Here's how the part is built. I have some questions about the finished solid (model axes, mm). A direction names the side the tool comes from. Coordinates: 2 decimals unless noted, no trailing zeros. Write each loop counter-clockwise with the first axis right and the second up, starting at its lowest first coordinate (ties: lowest second). Pieces come first, ordered by that corner, then holes. Notation, with made-up numbers: (39, 26) -> (46, 26) arc R27 ccw to (46, 65) -> close; hole circle Ø7 at (35, 74). An arc over 180 degrees is marked (long way). Use a Markdown table: item, result. Add a question column.
```python
from build123d import *

# Parameters (mm, degrees)
BODY_DEPTH             = 10
SKETCH14_R             = 7.5
BEARING_SUPPORT_DEPTH  = 15
SKETCH15_R             = 7.5
SKETCH15_R_2           = 4.7
BEARING_PLACE_DEPTH    = 4
SKETCH16_R             = 2
MOTOR_SHAFT_HOLE_DEPTH = 3
FILLET1_R              = 6
SKETCH17_R             = 7.25
SPRING_HOLE_DEPTH      = 10
SKETCH18_W             = 11
SKETCH18_H             = 6
NUT_HOLE_DEPTH         = 20
SKETCH19_R             = 3.25
SHAFT_HOLE_DEPTH       = 13
SKETCH20_R             = 3.25
BRAKE_DISK_HOLES_DEPTH = 67.708320321


with BuildPart() as part:
    # Sketch1 → Body (new, symmetric)
    with BuildSketch(Plane.XY):
        Polygon((-25, 25), (-15, 45), (15, 45), (25, 25), (25, 5), (45, 5), (45, -25), (25, -25), (-25, -25), (-45, -25), (-45, 5), (-25, 5), align=None)
    extrude(amount=BODY_DEPTH, both=True)

    # Sketch14 → Bearing_Support (add)
    with BuildSketch(Plane(origin=(0, 0, -10), x_dir=(-1, 0, 0), z_dir=(0, 0, -1))):
        Circle(SKETCH14_R)
    extrude(amount=BEARING_SUPPORT_DEPTH)

    # Sketch15 → Bearing_Place (add)
    with BuildSketch(Plane(origin=(0, 0, -25), x_dir=(-1, 0, 0), z_dir=(0, 0, -1))):
        Circle(SKETCH15_R)
        Circle(SKETCH15_R_2, mode=Mode.SUBTRACT)
    extrude(amount=BEARING_PLACE_DEPTH)

    # Sketch16 → Motor_Shaft_Hole (cut)
    with BuildSketch(Plane(origin=(0, 0, -25), x_dir=(-1, 0, 0), z_dir=(0, 0, -1))):
        Circle(SKETCH16_R)
    extrude(amount=-MOTOR_SHAFT_HOLE_DEPTH, mode=Mode.SUBTRACT)

    # Fillet1
    fillet1_edges = [part.edges().sort_by_distance(p)[0] for p in [
        (7.5, 0, -10),
    ]]
    fillet(fillet1_edges, radius=FILLET1_R)

    # Sketch17 → Spring_Hole (cut)
    with BuildSketch(Plane(origin=(0, 5, 0), x_dir=(1, 0, 0), z_dir=(0, 1, 0))):
        with Locations(Location((-35, 0, 0), (0, 0, 180))):
            Circle(SKETCH17_R)
    spring_hole = extrude(amount=-SPRING_HOLE_DEPTH, mode=Mode.SUBTRACT)

    # Sketch18 → Nut_Hole (cut)
    with BuildSketch(Plane.ZY.offset(45)):
        with Locations((0, -15)):
            Rectangle(SKETCH18_W, SKETCH18_H)
    nut_hole = extrude(amount=-NUT_HOLE_DEPTH, mode=Mode.SUBTRACT)

    # Sketch19 → Shaft_Hole (cut)
    with BuildSketch(Plane(origin=(0, -5, 0), x_dir=(1, 0, 0), z_dir=(0, 1, 0))):
        with Locations(Location((-35, 0, 0), (0, 0, 180))):
            Circle(SKETCH19_R)
    shaft_hole = extrude(amount=-SHAFT_HOLE_DEPTH, mode=Mode.SUBTRACT)

    # Mirror1: Spring_Hole, Nut_Hole, Shaft_Hole across plane
    add(spring_hole.mirror(Plane(origin=(0, 0, 0), x_dir=(0, 0, 1), z_dir=(1, 0, 0))), mode=Mode.SUBTRACT)
    add(nut_hole.mirror(Plane(origin=(0, 0, 0), x_dir=(0, 0, 1), z_dir=(1, 0, 0))), mode=Mode.SUBTRACT)
    add(shaft_hole.mirror(Plane(origin=(0, 0, 0), x_dir=(0, 0, 1), z_dir=(1, 0, 0))), mode=Mode.SUBTRACT)

    # Sketch20 → Brake_Disk_Holes (cut, through all)
    with BuildSketch(Plane(origin=(0, 0, -10), x_dir=(-1, 0, 0), z_dir=(0, 0, -1))):
        with Locations((-5.98239088, 24.273668848)):
            Circle(SKETCH20_R)
        with Locations((24.012809306, -6.955931947)):
            Circle(SKETCH20_R)
        with Locations((-18.030418426, -17.317736902)):
            Circle(SKETCH20_R)
    extrude(amount=-BRAKE_DISK_HOLES_DEPTH, mode=Mode.SUBTRACT)


solid = part.part
```
Q1. Which directions (+Z, -Z, +X, -X, +Y, -Y) give clear straight access to the entire face, cutting with the end or side of a thin tool? Please do faces 3 (the cylindrical face through (38.002, -8.451, -1.245)), 4 (the cylindrical face through (7.493, 0.33, -22.409)), 5 (the flat face through (35, -15, -5.5)), 6 (the flat face through (28, 5, 5)), 7 (the flat face through (-37, -12, -3)).
Q2. Please list where these lines run through material, in increasing order: line 1 (X direction, y = 2, z = 0.5); line 2 (Z direction, x = 35, y = 1.5); line 3 (Y direction, x = 29.5, z = -5).
Q3. Suppose I cut it at D-D, the plane z = 0. State how many separate pieces and enclosed holes the cut face has, and give its area (3 significant figures).
Q4. Suppose I cut it at B-B, the plane y = 0. Write out the boundary of the cut face in (x, z), and give its area (3 significant figures).
Q5. Suppose I cut it at C-C, the plane x = 35. Write out the boundary of the cut face in (y, z), and give its area (4 significant figures).
Q6. Suppose I cut it at A-A, the plane x = -22.5. Write out the boundary of the cut face in (y, z).
Q7. Thinking about a two-plate mould opening in Z: for faces 1 (the cylindrical face through (0, -2, -24)), 2 (the flat face through (35, -15, 5.5)), which applies, released by +Z, released by -Z, zero draft, split by the parting line, or undercut?
Q8. Will these pins go through, and if not, where does the flat tip stop? pin 1 (6 mm diameter, centred on y = 5.5, z = -24.5, fed in from +X); pin 2 (11.5 mm diameter, centred on x = -35, z = 0, fed in from +Y); pin 3 (11.5 mm diameter, centred on x = -37, z = 0, fed in from +Y); pin 4 (5 mm diameter, centred on x = 5.98, y = 24.27, fed in from +Z).
Answer key:
| question | item | result |
|---|---|---|
| 1 | face 3 | +Y |
| 1 | face 4 | -Z |
| 1 | face 5 | +X |
| 1 | face 6 | +Z, -Z, +X, +Y |
| 1 | face 7 | -X |
| 2 | line 1 | x = -45 to -42.23, -27.77 to 27.77, 42.23 to 45 |
| 2 | line 2 | z = -10 to -7.25, 7.25 to 10 |
| 2 | line 3 | y = -25 to -18, -12 to 5 |
| 3 | separate pieces | 3 |
| 3 | enclosed holes | 3 |
| 3 | area | 3,780 mm^2 |
| 4 | outline | (-45, -10) -> (-13.5, -10) arc R6 cw to (-7.5, -16) -> (-7.5, -29) -> (-4.7, -29) -> (-4.7, -25) -> (-2, -25) -> (-2, -22) -> (2, -22) -> (2, -25) -> (4.7, -25) -> (4.7, -29) -> (7.5, -29) -> (7.5, -16) arc R6 cw to (13.5, -10) -> (45, -10) -> (45, 10) -> (-45, 10) -> close; hole circle Ø14.5 at (-35, 0); hole circle Ø14.5 at (35, 0) |
| 4 | area | 1,720 mm^2 |
| 5 | outline | (-25, -10) -> (5, -10) -> (5, -7.25) -> (-5, -7.25) -> (-5, -3.25) -> (-12, -3.25) -> (-12, -5.5) -> (-18, -5.5) -> (-18, 5.5) -> (-12, 5.5) -> (-12, 3.25) -> (-5, 3.25) -> (-5, 7.25) -> (5, 7.25) -> (5, 10) -> (-25, 10) -> close |
| 5 | area | 343.5 mm^2 |
| 6 | outline | (-25, -10) -> (-9.83, -10) -> (-9.83, 10) -> (-25, 10) -> close; (-4.08, -10) -> (30, -10) -> (30, 10) -> (-4.08, 10) -> close |
| 7 | face 1 | zero draft |
| 7 | face 2 | undercut |
| 8 | pin 1 | stops at x = 7.07 |
| 8 | pin 2 | stops at y = -5 |
| 8 | pin 3 | stops at y = 5 |
| 8 | pin 4 | passes through |
